from build123d import *

# Parameters (mm, degrees)
ESBO_O1_R                = 7.5
RESSALTO_EXTRUS_O1_DEPTH = 5
CORTE_EXTRUS_O1_DEPTH    = 5
PADR_OCIRCULAR2_COUNT    = 14
ESBO_O2_R                = 25
ESBO_O2_R_2              = 5
RESSALTO_EXTRUS_O2_DEPTH = 2


with BuildPart() as part:
    # Esbo_o1 → Ressalto-extrus_o1 (new body)
    # profile 1 of 2: a face of its own
    with BuildSketch(Plane.XY):
        Circle(ESBO_O1_R)
        with BuildLine():
            ThreePointArc((-0.89, 6.438780941), (0, 6.5), (0.89, 6.438780941))
            Line((0.89, 6.438780941), (0.9, 4.816637832))
            ThreePointArc((0.9, 4.816637832), (3.769615365, 3.130495168), (4.9, 0))
            ThreePointArc((4.9, 0), (-3.130495168, -3.769615365), (-0.9, 4.816637832))
            Line((-0.9, 4.816637832), (-0.89, 6.438780941))
        make_face(mode=Mode.SUBTRACT)
    # profile 2 of 2: a face of its own
    with BuildSketch(Plane.XY):
        with BuildLine():
            Line((0.9, 4.816637832), (0.89, 6.438780941))
            ThreePointArc((0.89, 6.438780941), (0, 6.5), (-0.89, 6.438780941))
            Line((-0.89, 6.438780941), (-0.9, 4.816637832))
            ThreePointArc((-0.9, 4.816637832), (0, 4.9), (0.9, 4.816637832))
        make_face()
    extrude(amount=RESSALTO_EXTRUS_O1_DEPTH)

    # Esbo_o1_3 → Corte-extrus_o1 (cut)
    with BuildSketch(Plane.XY):
        with BuildLine():
            Line((0.9, 4.816637832), (0.89, 6.438780941))
            ThreePointArc((0.89, 6.438780941), (0, 6.5), (-0.89, 6.438780941))
            Line((-0.89, 6.438780941), (-0.9, 4.816637832))
            ThreePointArc((-0.9, 4.816637832), (0, 4.9), (0.9, 4.816637832))
        make_face()
    corte_extrus_o1 = extrude(amount=CORTE_EXTRUS_O1_DEPTH, mode=Mode.SUBTRACT)

    # Padr_oCircular2: Corte-extrus_o1 ×14 about axis
    padr_ocircular2_axis = Axis((0, 0, 0), (0, 0, 1))
    for i in range(1, PADR_OCIRCULAR2_COUNT):
        add(corte_extrus_o1.rotate(padr_ocircular2_axis, i * 360 / PADR_OCIRCULAR2_COUNT), mode=Mode.SUBTRACT)

    # Esbo_o2 → Ressalto-extrus_o2 (add)
    with BuildSketch(Plane.XY.offset(5)):
        Circle(ESBO_O2_R)
        with Locations((0, 16.25)):
            Circle(ESBO_O2_R_2, mode=Mode.SUBTRACT)
        with Locations((11.490485194, 11.490485194)):
            Circle(ESBO_O2_R_2, mode=Mode.SUBTRACT)
        with Locations((16.25, 0)):
            Circle(ESBO_O2_R_2, mode=Mode.SUBTRACT)
        with Locations((11.490485194, -11.490485194)):
            Circle(ESBO_O2_R_2, mode=Mode.SUBTRACT)
        with Locations((0, -16.25)):
            Circle(ESBO_O2_R_2, mode=Mode.SUBTRACT)
        with Locations((-11.490485194, -11.490485194)):
            Circle(ESBO_O2_R_2, mode=Mode.SUBTRACT)
        with Locations((-16.25, 0)):
            Circle(ESBO_O2_R_2, mode=Mode.SUBTRACT)
        with Locations((-11.490485194, 11.490485194)):
            Circle(ESBO_O2_R_2, mode=Mode.SUBTRACT)
    extrude(amount=RESSALTO_EXTRUS_O2_DEPTH)


solid = part.part
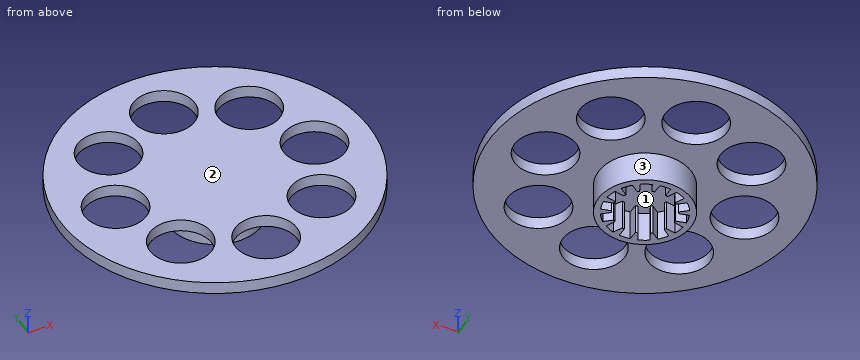
Build history of the part. All positions in model axes, mm. Face numbers are marked on the shaded views. Round coordinates to 2 decimals unless told otherwise and drop trailing zeros. Write each loop counter-clockwise with the first axis right and the second up, starting at its lowest first coordinate (ties: lowest second). Pieces come first, ordered by that corner, then holes. Notation, with made-up numbers: M 36,-39 L 50,-39 A21 ccw 50,-18 Z; hole C 8,44 d3. An arc over 180 degrees is marked long. Answer in a Markdown table with one row per item.
1. Saw through at B-B (y = 20). List the corners of the cut face in (x, z), and give its area (3 significant figures).
Geometry check:
| item | result |
|---|---|
| outline | M -15,5 L -3.31,5 L -3.31,7 L -15,7 Z; M 3.31,5 L 15,5 L 15,7 L 3.31,7 Z |
| area | 46.8 mm2 |
2. Saw through at A-A (x = 9). List the corners of the cut face in (y, z).
Geometry check:
| item | result |
|---|---|
| outline | M -23.32,5 L -15.83,5 L -15.83,7 L -23.32,7 Z; M -7.15,5 L 7.15,5 L 7.15,7 L -7.15,7 Z; M 15.83,5 L 23.32,5 L 23.32,7 L 15.83,7 Z |
3. Flat gauge pins, fed straight in: P1, Ø3, axis at x = 4.5, z = 6, coming from the -Y side; P2, Ø16, axis at x = 16.25, y = 0, coming from the -Z side; P3, Ø3, axis at y = 4, z = 4.5, coming from the +X side. Where does each tip first touch, or does it go through?
Geometry check:
| item | result |
|---|---|
| P1 | y = -24.82 |
| P2 | z = 5 |
| P3 | x = 24.87 |
4. Saw through at C-C (z = 5.75). State how many separate pieces and enclosed holes the cut face has, and give its area (3 significant figures).
Geometry check:
| item | result |
|---|---|
| separate pieces | 1 |
| enclosed holes | 8 |
| area | 1,340 mm2 |
5. Mould opens along X. For the marked faces 1, 2 and 3 say: +X half, -X half, draft (parallel to the pull), parting line (faces both ways), or undercut.
Geometry check:
| item | result |
|---|---|
| face 1 | undercut |
| face 2 | draft |
| face 3 | parting line |
6. Saw through at D-D (x = 19.5). List the corners of the cut face in (y, z).
Geometry check:
| item | result |
|---|---|
| outline | M -15.64,5 L -3.8,5 L -3.8,7 L -15.64,7 Z; M 3.8,5 L 15.64,5 L 15.64,7 L 3.8,7 Z |
7. Probe L1, parallel to Y at x = 0, z = 5.8; L2, parallel to X at y = 9, z = 5.5; L3, parallel to X at y = -3, z = 6. List the from-to ranges inside material, lowest first. Write a range as [from, to].
Geometry check:
| item | result |
|---|---|
| L1 | [-25, -21.25], [-11.25, 11.25], [21.25, 25] |
| L2 | [-23.32, -15.83], [-7.15, 7.15], [15.83, 23.32] |
| L3 | [-24.82, -20.25], [-12.25, 12.25], [20.25, 24.82] |
